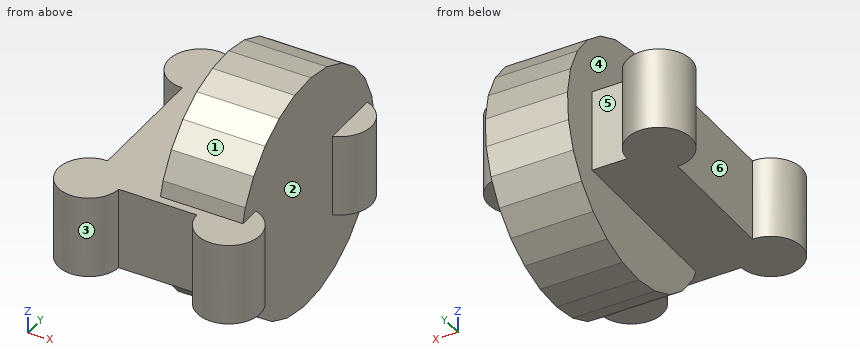
from build123d import *

# Parameters (mm, degrees)
F0_W     = 42.961035
F0_H     = 59.7119
F1_DEPTH = 25.4
F2_R     = 9.839641
F2_R_2   = 9.85345
F2_R_3   = 9.734491
F2_R_4   = 9.512534
F3_DEPTH = 25.4
F5_DEPTH = 25.4


with BuildPart() as f1:
    # F0 (on Top) → F1 (new body)
    with BuildSketch(Plane.XY):
        with Locations((0.788275, -6.995948)):
            Rectangle(F0_W, F0_H)
    extrude(amount=F1_DEPTH)

    # F2 (on Top) → F3 (join)
    with BuildSketch(Plane.XY):
        with Locations((22.268793, 22.66293)):
            Circle(F2_R)
        with Locations((-20.692242, 22.860002)):
            Circle(F2_R_2)
        with Locations((22.465866, -36.654826)):
            Circle(F2_R_3)
        with Locations((-20.889312, -36.260691)):
            Circle(F2_R_4)
    extrude(amount=F3_DEPTH)

    # F4 (on Right) → F5 (join)
    with BuildSketch(Plane.YZ):
        Polygon((-1.96623, -20.782315), (6.695889, -20.20803), (14.968867, -17.577453), (22.371909, -13.043462), (28.474777, -6.869556), (32.922794, 0.585458), (35.457458, 8.888324), (35.931464, 17.556509), (34.317264, 26.086249), (30.708669, 33.981826), (25.315398, 40.784379), (18.450887, 46.098569), (10.514079, 49.615552), (1.96623, 51.130936), (-6.695889, 50.556652), (-14.968867, 47.926074), (-22.371909, 43.392083), (-28.474777, 37.218178), (-32.922794, 29.763163), (-35.457458, 21.460297), (-35.931464, 12.792113), (-34.317264, 4.262373), (-30.708669, -3.633205), (-25.315398, -10.435758), (-18.450887, -15.749947), (-10.514079, -19.266931), align=None)
    extrude(amount=F5_DEPTH)


solid = f1.part
Can you work these out from the model? Positions are in its coordinate system, mm. Face numbers are marked on the shaded views. A direction names the side the tool comes from. Give positions to 0.01 mm unless a question says otherwise; leave off trailing zeros. Loops run counter-clockwise (first coordinate to the right, second up) from the corner with the lowest first, then second, coordinate; pieces in that order, holes last. Notation, with made-up numbers: (80.5, -40) -> (132.5, -40) arc R15 ccw to (132.5, -36) -> close; hole circle Ø5 at (37.25, -37.5). An arc over 180 degrees is marked (long way). Return JSON: item names as keys, results as strings.
Q1. I want a section at A-A, the plane x = -26.5. List the corners of the cut face in (y, z) for me, then the cut area to 3 significant figures.
Checks:
{"outline": "(-43.94, 0) -> (-28.58, 0) -> (-28.58, 25.4) -> (-43.94, 25.4) -> close; (14.9, 0) -> (30.82, 0) -> (30.82, 25.4) -> (14.9, 25.4) -> close", "area": "795 mm2"}
Q2. For pin 1 Ø7.5 at (x, y) = (27.5, 25) entering from +Z; pin 2 Ø12 at (x, z) = (26, 28) entering from -Y; pin 3 Ø6 at (x, z) = (-5, -1) entering from -Y; pin 4 Ø2 at (x, y) = (30, 26) entering from -Z, each with a flat end and sliding along its axis, tell me the tip position at first contact or that it passes through.
Checks:
{"pin 1": "stops at z = 43.43", "pin 2": "stops at y = -46.39", "pin 3": "stops at y = -36.85", "pin 4": "stops at z = 0"}
Q3. I want a section at C-C, the plane z = 13.5. List the corners of the cut face in (x, y) for me, then the cut area to 3 significant figures.
Checks:
{"outline": "(-20.69, -26.75) arc R9.51 ccw (long way) to (-11.4, -36.85) -> (12.73, -36.85) arc R9.73 ccw (long way) to (25.4, -27.37) -> (25.4, 13.33) arc R9.84 ccw to (25.4, 31.99) -> (25.4, 35.71) -> (0, 35.71) -> (0, 22.86) -> (-10.84, 22.86) arc R9.85 ccw (long way) to (-20.69, 13.01) -> close", "area": "3,800 mm2"}
Q4. I need wall thicknesses on probe 1 along X at (y, z) = (-2, 19.5); probe 2 along Z at (x, y) = (-8, 15). Which ranges of each line are inside material? Lowest first, please.
Checks:
{"probe 1": "x = -20.69 to 25.4", "probe 2": "z = 0 to 25.4"}
Q5. I want a section at B-B, the plane x = 4.5. List the corners of the cut face in (y, z) for me.
Checks:
{"outline": "(-36.85, 0) -> (-32.37, 0) -> (-30.71, -3.63) -> (-25.32, -10.44) -> (-18.45, -15.75) -> (-10.51, -19.27) -> (-1.97, -20.78) -> (6.7, -20.21) -> (14.97, -17.58) -> (22.37, -13.04) -> (28.47, -6.87) -> (32.92, 0.59) -> (35.46, 8.89) -> (35.93, 17.56) -> (34.32, 26.09) -> (30.71, 33.98) -> (25.32, 40.78) -> (18.45, 46.1) -> (10.51, 49.62) -> (1.97, 51.13) -> (-6.7, 50.56) -> (-14.97, 47.93) -> (-22.37, 43.39) -> (-28.47, 37.22) -> (-32.92, 29.76) -> (-34.25, 25.4) -> (-36.85, 25.4) -> close"}
Q6. We'd pull the mould along X, two halves only. Please class the marked faces 1, 2 and 3: released by +X, released by -X, zero draft, split by the parting line, or undercut.
Checks:
{"face 1": "zero draft", "face 2": "released by +X", "face 3": "undercut"}
Q7. I want a section at D-D, the plane y = 5. List the corners of the cut face in (x, z) for me, then the cut area to 3 significant figures.
Checks:
{"outline": "(-20.69, 0) -> (0, 0) -> (0, -20.32) -> (25.4, -20.32) -> (25.4, 50.59) -> (0, 50.59) -> (0, 25.4) -> (-20.69, 25.4) -> close", "area": "2,330 mm2"}
Q8. On a 3-axis mill with a long thin cutter (end or side, diameter ignored), from which of +Z, -Z, +X, -X, +Y, -Y can I reach the whole of each face in a straight line? I mean the marked faces 4, 5 and 6. Say none if no direction works.
Checks:
{"face 4": "+Y", "face 5": "+Z, -Z, +Y", "face 6": "+Z, -Z, -X"}
